Here's how the part is built. I have some questions about the finished solid (model axes, mm). A direction names the side the tool comes from. Coordinates: 2 decimals unless noted, no trailing zeros. Order: outer loops, then holes, each group sorted by start corner. A loop starts at its lowest first (then second) coordinate and runs counter-clockwise, first axis right, second up. Notation, with made-up numbers: (71.25, 82.25) - (101.25, 82.25) arc R25 cw to (101.25, 121.25) - close; hole circle Ø11 at (15, 26). An arc over 180 degrees is marked (long way). Answer as CSV lines item,"result". Start each with the question number.
Q1. Suppose I cut it at B-B (x = 2). Please give me the cut outline in (y, z).
Q2. I need wall thicknesses on line 1 (X direction, y = -13, z = 4); line 2 (X direction, y = 17, z = 23.5); line 3 (X direction, y = -7.5, z = 4.25). Which ranges of each line are inside material? Lowest first, please.
Q3. Suppose I cut it at C-C (y = -14). Please give me the cut outline in (x, z), then the cut area to 3 significant figures.
Q4. Suppose I cut it at A-A (z = 28.25). Please give me the cut outline in (x, y), then the cut area to 3 significant figures.
Q5. For pin 1 Ø1.5 at (x, z) = (-24.5, 13) entering from -Y; pin 2 Ø2 at (y, z) = (16, 19) entering from +X; pin 3 Ø3 at (x, z) = (-3.5, 19.5) entering from +Y, each with a flat end and sliding along its axis, tell me the tip position at first contact or that it passes through.
Q6. For faces 4 (the face through (0, 13, 15)), 5 (the face through (-25, -3, 15)), 6 (the face through (22.5, -12, 15)), 7 (the face through (-9.75, -18, 7)), which set-ups out of +Z, -Z, +X, -X, +Y, -Y let a thin tool reach every point of the face, with its end or its side?
Q7. Suppose I cut it at D-D (z = 12.75). Please give me the cut outline in (x, y), then the cut area to 3 significant figures.
Q8. Thinking about a two-plate mould opening in X: for faces 1 (the face through (0.136, -15.437, 12.818)), 2 (the face through (16, 20, 15)), 3 (the face through (-22.5, -11, 15)), which applies, released by +X, released by -X, zero draft, split by the parting line, or undercut?
from build123d import *

# Parameters (mm, degrees)
EXTRUDE_1_DEPTH                 = 30
CUT_EXTRUDE_1_REACH             = 47.346
CUT_EXTRUDE_1_DIRECTION_2_REACH = 47.346


with BuildPart() as part:
    # Эскиз1 → Бобышка-Вытянуть1 (new body)
    with BuildSketch(Plane.XY):
        Polygon((-22.5, -3), (-22.5, -20), (22.5, -20), (22.5, -3), (27.5, -3), (27.5, 13), (22.5, 13), (22.5, 20), (9.75, 20), (9.75, 13), (-9.75, 13), (-9.75, 20), (-27.5, 20), (-27.5, -3), align=None)
    extrude(amount=EXTRUDE_1_DEPTH)

    # Вырез-Вытянуть1: up to this face of the body (flat: up to its plane)
    cut_extrude_1_end = Plane(part.part.faces().sort_by_distance((-9.75, 16.5, 15))[0])
    # Эскиз2 → Вырез-Вытянуть1 (cut, up to the picked face)
    with BuildSketch(Plane(origin=(0, 0, 0), x_dir=(0, 0, -1), z_dir=(1, 0, 0)), mode=Mode.PRIVATE) as cut_extrude_1_sk1:
        Polygon((0, -20), (0, -11), (-26, -20), align=None)
    cut_extrude_1_tool1 = split(extrude(cut_extrude_1_sk1.sketch, amount=-CUT_EXTRUDE_1_REACH, mode=Mode.PRIVATE), bisect_by=cut_extrude_1_end, keep=Keep.BOTH, mode=Mode.PRIVATE)
    add(cut_extrude_1_tool1.solids().sort_by(Axis((0, -17, 8.666667), (-1, 0, 0)))[0], mode=Mode.SUBTRACT)

    # Вырез-Вытянуть1 direction 2: up to this face of the body (flat: up to its plane)
    cut_extrude_1_direction_2_end = Plane(part.part.faces().sort_by_distance((9.75, 16.5, 15))[0])
    # Эскиз2 → Вырез-Вытянуть1 direction 2 (cut, up to the picked face)
    with BuildSketch(Plane(origin=(0, 0, 0), x_dir=(0, 0, -1), z_dir=(1, 0, 0)), mode=Mode.PRIVATE) as cut_extrude_1_direction_2_sk1:
        Polygon((0, -20), (0, -11), (-26, -20), align=None)
    cut_extrude_1_direction_2_tool1 = split(extrude(cut_extrude_1_direction_2_sk1.sketch, amount=CUT_EXTRUDE_1_DIRECTION_2_REACH, mode=Mode.PRIVATE), bisect_by=cut_extrude_1_direction_2_end, keep=Keep.BOTH, mode=Mode.PRIVATE)
    add(cut_extrude_1_direction_2_tool1.solids().sort_by(Axis((0, -17, 8.666667), (1, 0, 0)))[0], mode=Mode.SUBTRACT)


solid = part.part
Here are the results:
1,outline,"(-20, 26) - (-11, 0) - (13, 0) - (13, 30) - (-20, 30) - close"
2,line 1,"x = -22.5 to -9.75, 9.75 to 22.5"
2,line 2,"x = -27.5 to -9.75, 9.75 to 22.5"
2,line 3,"x = -22.5 to 22.5"
3,outline,"(-22.5, 0) - (-9.75, 0) - (-9.75, 8.67) - (9.75, 8.67) - (9.75, 0) - (22.5, 0) - (22.5, 30) - (-22.5, 30) - close"
3,area,"1,180 mm²"
4,outline,"(-27.5, -3) - (-22.5, -3) - (-22.5, -20) - (22.5, -20) - (22.5, -3) - (27.5, -3) - (27.5, 13) - (22.5, 13) - (22.5, 20) - (9.75, 20) - (9.75, 13) - (-9.75, 13) - (-9.75, 20) - (-27.5, 20) - close"
4,area,"1,860 mm²"
5,pin 1,"stops at y = -3"
5,pin 2,"stops at x = 22.5"
5,pin 3,"stops at y = 13"
6,face 4,"+Z, -Z, +Y"
6,face 5,"+Z, -Z, -X, -Y"
6,face 6,"+Z, -Z, +X, -Y"
6,face 7,"-Z, -Y"
7,outline,"(-27.5, -3) - (-22.5, -3) - (-22.5, -20) - (-9.75, -20) - (-9.75, -15.41) - (9.75, -15.41) - (9.75, -20) - (22.5, -20) - (22.5, -3) - (27.5, -3) - (27.5, 13) - (22.5, 13) - (22.5, 20) - (9.75, 20) - (9.75, 13) - (-9.75, 13) - (-9.75, 20) - (-27.5, 20) - close"
7,area,"1,770 mm²"
8,face 1,"undercut"
8,face 2,"zero draft"
8,face 3,"released by -X"
